Read the model definition and answer for the solid it produces. Units are mm, in the model's axes. A direction names the side the tool comes from. Give positions to 0.01 mm unless a question says otherwise; leave off trailing zeros. Loops run counter-clockwise (first coordinate to the right, second up) from the corner with the lowest first, then second, coordinate; pieces in that order, holes last. Notation, with made-up numbers: (7.25, -33.75) - (35.25, -33.75) arc R33 ccw to (35.25, -0.75) - close; hole circle Ø7 at (-2, 69.5). An arc over 180 degrees is marked (long way). Write each question's results on one line, items separated by ' | '. Start each with the question number.
Q1. For faces 1 (the flat face through (0, -2, -11.5)), 2 (the flat face through (-59, -7, 0)), 3 (the flat face through (-46, -6, 4)), 4 (the flat face through (71, -7, 0)), 5 (the cylindrical face through (-77.488, -2.958, 0.55)), determine the directions among +Z, -Z, +X, -X, +Y, -Y from which every point of the face is accessible in a straight line to the end or side of a thin tool.
Q2. Determine the mould class of faces 6 (the cylindrical face through (-78.487, -3.958, 0.594)), 7 (the flat face through (-1, 0, 0)), 8 (the cylindrical face through (55.08, -2.958, -7.606)) for opening direction X: +X half, -X half, draft (parallel to the pull), parting line (faces both ways), or undercut.
Q3. Find the intervals of material crossed by line 1 (X direction, y = -9, z = 18); line 2 (Y direction, x = 28, z = -6); line 3 (Z direction, x = 65, y = -6.55), in increasing order. Write a range as from..to.
Q4. The part is cut by section C-C, the plane z = 19. Write down the section's boundary in (x, y).
Q5. The part is cut by section A-A, the plane y = -15. Write down the section's boundary in (x, z).
Q6. Given pin 1 (3.5 mm diameter, centred on x = -7, y = -4.5, fed in from -Z); pin 2 (3 mm diameter, centred on x = -5.5, z = -14, fed in from -Y); pin 3 (11 mm diameter, centred on y = -36, z = -1.5, fed in from -X), each flat-ended and moving along its own axis, determine where each tip first touches the part or whether it passes through.
Q7. The part is cut by section B-B, the plane x = -26.5. Write down the section's boundary in (y, z), plus the area to 3 significant figures.
```python
from build123d import *

# Parameters (mm, degrees)
F0_W      = 165
F0_H      = 45
F0_R      = 12.5
F1_DEPTH  = 1
F3_DEPTH  = 1
F4_DEPTH  = 25
F5_DEPTH  = 25
F6_R      = 13.5
F6_R_2    = 12.5
F7_DEPTH  = 5
F8_R      = 13.5
F8_R_2    = 5
F9_DEPTH  = 1
F11_DEPTH = 1
F12_W     = 1
F12_H     = 1
F12_H_2   = 36
F12_W_2   = 92
F13_DEPTH = 11
F14_W     = 94
F14_H     = 37
F15_DEPTH = 1
F16_W     = 1
F16_H     = 36
F17_DEPTH = 66
F18_W     = 26.2803444985
F18_H     = 1
F19_DEPTH = 3


with BuildPart() as f1:
    # F0 (on Front) → F1 (new body)
    with BuildSketch(Plane.XZ):
        Rectangle(F0_W, F0_H)
        with Locations((-65, 0)):
            Circle(F0_R, mode=Mode.SUBTRACT)
        with Locations((65, 0)):
            Circle(F0_R, mode=Mode.SUBTRACT)
    extrude(amount=F1_DEPTH)

    # F2 (on face) → F3 (join)
    with BuildSketch(Plane.XZ.offset(1)):
        with BuildLine():
            Line((68.3925151825, -19.0988145769), (65, -22.5))
            ThreePointArc((65, -22.5), (87.5, 0), (65, 22.5))
            Line((65, 22.5), (71.474224329, 16.2770561874))
            Line((71.474224329, 16.2770561874), (77.4062722921, 9.1145541519))
            Line((77.4062722921, 9.1145541519), (80.3926512599, 2.1407562308))
            Line((80.3926512599, 2.1407562308), (80.3926512599, -5.2317115478))
            Line((80.3926512599, -5.2317115478), (78.3914923668, -12.1520543471))
            Line((78.3914923668, -12.1520543471), (74.6632069349, -14.4081749022))
            Line((74.6632069349, -14.4081749022), (68.3925151825, -19.0988145769))
        make_face()
        with BuildLine():
            Line((-65, 14.9617949501), (-65, 22.5))
            ThreePointArc((-65, 22.5), (-87.5, 0), (-65, -22.5))
            Line((-65, -22.5), (-67.4760043621, -15.6979020685))
            Line((-67.4760043621, -15.6979020685), (-72.8440880775, -12.9142012447))
            Line((-72.8440880775, -12.9142012447), (-76.5851810575, -7.8018400818))
            Line((-76.5851810575, -7.8018400818), (-79.5639529824, 0))
            Line((-79.5639529824, 0), (-79.5639529824, 6.4657721668))
            Line((-79.5639529824, 6.4657721668), (-75.4495188594, 11.7608513683))
            Line((-75.4495188594, 11.7608513683), (-65, 14.9617949501))
        make_face()
    extrude(amount=-F3_DEPTH)

    # F2 (on face) → F4 (cut)
    with BuildSketch(Plane.XZ.offset(1)):
        with BuildLine():
            Line((-82.5, 22.5), (-82.5, 14.1421356237))
            ThreePointArc((-82.5, 14.1421356237), (-74.6966991411, 20.3033008589), (-65, 22.5))
            Line((-65, 22.5), (-82.5, 22.5))
        make_face()
    extrude(amount=-F4_DEPTH, mode=Mode.SUBTRACT)

    # F2 (on face) → F5 (cut)
    with BuildSketch(Plane.XZ.offset(1)):
        with BuildLine():
            ThreePointArc((82.5, -14.1421356237), (74.6966991411, -20.3033008589), (65, -22.5))
            Line((65, -22.5), (82.5, -22.5))
            Line((82.5, -22.5), (82.5, -14.1421356237))
        make_face()
        with BuildLine():
            ThreePointArc((65, 22.5), (74.6966991411, 20.3033008589), (82.5, 14.1421356237))
            Line((82.5, 14.1421356237), (82.5, 22.5))
            Line((82.5, 22.5), (65, 22.5))
        make_face()
        with BuildLine():
            Line((-82.5, -22.5), (-65, -22.5))
            ThreePointArc((-65, -22.5), (-74.6966991411, -20.3033008589), (-82.5, -14.1421356237))
            Line((-82.5, -14.1421356237), (-82.5, -22.5))
        make_face()
    extrude(amount=-F5_DEPTH, mode=Mode.SUBTRACT)

    # F6 (on face) → F7 (join)
    with BuildSketch(Plane.XZ.offset(1)):
        with Locations((-65, 0)):
            Circle(F6_R)
        with Locations((-65, 0)):
            Circle(F6_R_2, mode=Mode.SUBTRACT)
        with Locations((65, 0)):
            Circle(F6_R)
        with Locations((65, 0)):
            Circle(F6_R_2, mode=Mode.SUBTRACT)
    extrude(amount=F7_DEPTH)

    # F8 (on face) → F9 (join)
    with BuildSketch(Plane.XZ.offset(6)):
        with Locations((-65, 0)):
            Circle(F8_R)
        with Locations((-65, 0)):
            Circle(F8_R_2, mode=Mode.SUBTRACT)
        with Locations((65, 0)):
            Circle(F8_R)
        with Locations((65, 0)):
            Circle(F8_R_2, mode=Mode.SUBTRACT)
    extrude(amount=F9_DEPTH)

    # F10 (on face) → F11 (join)
    with BuildSketch(Plane.XZ.offset(1)):
        Polygon((-81.9395110011, 0), (-87.5, 0), (-87.5, -22.5), (-65, -22.5), (-65, -18.5897927731), (-73.3228996396, -16.0001199692), (-80.1934376359, -9.6208481118), align=None)
    extrude(amount=-F11_DEPTH)

    # F12 (on face) → F13 (join)
    with BuildSketch(Plane.XZ.offset(1)):
        with Locations((46.5, -14)):
            Rectangle(F12_W, F12_H)
        with Locations((46.5, 4.5)):
            Rectangle(F12_W, F12_H_2)
        with Locations((0, -14)):
            Rectangle(F12_W_2, F12_H)
        with Locations((-46.5, -14)):
            Rectangle(F12_W, F12_H)
        with Locations((-46.5, 4.5)):
            Rectangle(F12_W, F12_H_2)
    extrude(amount=F13_DEPTH)

    # F14 (on face) → F15 (join)
    with BuildSketch(Plane.XZ.offset(12)):
        with Locations((0, 4)):
            Rectangle(F14_W, F14_H)
    extrude(amount=F15_DEPTH)

    # F16 (on face) → F17 (join)
    with BuildSketch(Plane.XZ.offset(13)):
        with Locations((-46.5, 4.5)):
            Rectangle(F16_W, F16_H)
        with Locations((46.5, 4.5)):
            Rectangle(F16_W, F16_H)
    extrude(amount=F17_DEPTH)

    # F18 (on face) → F19 (join)
    with BuildSketch(Plane.XZ.offset(1)):
        with Locations((0.058112666, -11)):
            Rectangle(F18_W, F18_H)
    extrude(amount=F19_DEPTH)


solid = f1.part
```
Check sheet entries:
1) face 1: none | face 2: +Z, -Z, -X, -Y | face 3: +Z | face 4: +Z, -Z, +X, -Y | face 5: +Y
2) face 6: undercut | face 7: draft | face 8: undercut
3) line 1: x = -47..-46, 46..47 | line 2: y = -13..-12, -1..0 | line 3: z = -13.5..-5, 5..13.5
4) outline: (-77.05, -1) - (-47, -1) - (-47, -79) - (-46, -79) - (-46, -13) - (46, -13) - (46, -79) - (47, -79) - (47, -1) - (77.05, -1) - (77.05, 0) - (-77.05, 0) - close; hole (-46, -12) - (46, -12) - (46, -1) - (-46, -1) - close
5) outline: (-47, -13.5) - (-46, -13.5) - (-46, 22.5) - (-47, 22.5) - close; (46, -13.5) - (47, -13.5) - (47, 22.5) - (46, 22.5) - close
6) pin 1: stops at z = -14.5 | pin 2: stops at y = -13 | pin 3: stops at x = -47
7) outline: (-13, -14.5) - (-1, -14.5) - (-1, -22.5) - (0, -22.5) - (0, 22.5) - (-1, 22.5) - (-1, -13.5) - (-12, -13.5) - (-12, 22.5) - (-13, 22.5) - close | area: 93.0 mm^2
